Model file for the job. Use its own axes, mm. A direction names the side the tool comes from. Round coordinates to 2 decimals unless told otherwise and drop trailing zeros. Order: outer loops, then holes, each group sorted by start corner. A loop starts at its lowest first (then second) coordinate and runs counter-clockwise, first axis right, second up. Notation, with made-up numbers: (72, 9.25) - (119, 9.25) arc R33 ccw to (119, 47.25) - close; hole circle Ø7 at (-31, 27.25). An arc over 180 degrees is marked (long way). Use one line per item in the form item = value.
from build123d import *

# Parameters (mm, degrees)
F2_R     = 45.1358
F3_DEPTH = 20
F4_R     = 45.1358
F5_DEPTH = 20
F6_R     = 40
F7_DEPTH = 127


with BuildPart() as f1:
    # F0 (on Right) → F1 (revolve)
    with BuildSketch(Plane.YZ):
        Polygon((-46.0375, 0), (0, 0), (0, 50.8), (-39.6875, 103.1875), (-46.0375, 103.1875), align=None)
        Polygon((0, 0), (46.0375, 0), (46.0375, 103.1875), (39.6875, 103.1875), (0, 50.8), align=None)
    revolve(axis=Axis((0, 0, 0), (0, 1, 0)))

    # F2 (on face) → F3 (cut)
    with BuildSketch(Plane(origin=(0, 46.0375, 0), x_dir=(-1, 0, 0), z_dir=(0, 1, 0))):
        Circle(F2_R)
    extrude(amount=-F3_DEPTH, mode=Mode.SUBTRACT)

    # F4 (on face) → F5 (cut)
    with BuildSketch(Plane.XZ.offset(46.0375)):
        Circle(F4_R)
    extrude(amount=-F5_DEPTH, mode=Mode.SUBTRACT)

    # F6 (on face) → F7 (cut)
    with BuildSketch(Plane.XZ.offset(26.0375)):
        Circle(F6_R)
    extrude(amount=-F7_DEPTH, mode=Mode.SUBTRACT)


solid = f1.part
(1) Slice it at A-A on x = 0. Give the cut face in (y, z).
Report:
outline = (-46.04, -103.19) - (-39.69, -103.19) - (0, -50.8) - (39.69, -103.19) - (46.04, -103.19) - (46.04, -45.14) - (26.04, -45.14) - (26.04, -40) - (-26.04, -40) - (-26.04, -45.14) - (-46.04, -45.14) - close; (-46.04, 45.14) - (-26.04, 45.14) - (-26.04, 40) - (26.04, 40) - (26.04, 45.14) - (46.04, 45.14) - (46.04, 103.19) - (39.69, 103.19) - (0, 50.8) - (-39.69, 103.19) - (-46.04, 103.19) - close
(2) Slice it at C-C on y = -21. Give the cut face in (x, z), then the cut area to 3 significant figures.
Report:
outline = circle Ø157.04 at (0, 0); hole circle Ø80 at (0, 0)
area = 14,300 mm2
(3) Pin check, flat tips, straight feed: pin 1 (3 mm diameter, centred on x = -34.5, y = 33.5, fed in from -Z); pin 2 (10 mm diameter, centred on y = 11, z = 53.5, fed in from +X); pin 3 (10 mm diameter, centred on x = 68, y = 24.5, fed in from -Z). Stop position of each tip, or through.
Report:
pin_1 = -90.73
pin_2 = 49.45
pin_3 = -60.04
(4) Pull direction X, two halves, no side cores. Call faces 1 (the face through (4, 26.038, -40)), 2 (the face through (-62.788, -42.907, -81.886)), 3 (the face through (43.05, -36.18, 13.56)), 4 (the face through (-21, -46.038, 44)): released by +X, released by -X, zero draft, split by the parting line, or undercut.
Report:
face_1 = undercut
face_2 = split by the parting line
face_3 = undercut
face_4 = zero draft
(5) Probe probe 1 along Z at (x, y) = (0, 9); probe 2 along Y at (x, z) = (44.5, 3.5); probe 3 along X at (y, z) = (-34.5, 33). List the from-to ranges inside material, lowest first. Write a range as [from, to].
Report:
probe_1 = [-62.68, -40], [40, 62.68]
probe_2 = [-26.04, 26.04]
probe_3 = [-90.51, -30.79], [30.79, 90.51]
(6) Slice it at B-B on z = 0. Give the cut face in (x, y).
Report:
outline = (-103.19, -46.04) - (-45.14, -46.04) - (-45.14, -26.04) - (-40, -26.04) - (-40, 26.04) - (-45.14, 26.04) - (-45.14, 46.04) - (-103.19, 46.04) - (-103.19, 39.69) - (-50.8, 0) - (-103.19, -39.69) - close; (40, -26.04) - (45.14, -26.04) - (45.14, -46.04) - (103.19, -46.04) - (103.19, -39.69) - (50.8, 0) - (103.19, 39.69) - (103.19, 46.04) - (45.14, 46.04) - (45.14, 26.04) - (40, 26.04) - close
(7) Slice it at D-D on y = -5.5. Give the cut face in (x, z).
Report:
outline = circle Ø116.12 at (0, 0); hole circle Ø80 at (0, 0)
(8) Tool access for faces 5 (the face through (-47.976, -2.483, 24.953)), 6 (the face through (-21, 46.038, -44)), 7 (the face through (-4, -26.038, -40)), 8 (the face through (-8.67, -0.36, -39.05)), 9 (the face through (-43.05, 36.18, 13.56)): list every direction of +Z, -Z, +X, -X, +Y, -Y with a clear straight run to the whole face (end or side of a thin tool).
Report:
face_5 = none
face_6 = +Z, -Z, +X, -X, +Y
face_7 = -Y
face_8 = +Y, -Y
face_9 = +Y
